The listing builds one solid part. Answer for the finished solid, in the listing's coordinates (mm). A direction names the side the tool comes from. Coordinates: 2 decimals unless noted, no trailing zeros. Loops run counter-clockwise (first coordinate to the right, second up) from the corner with the lowest first, then second, coordinate; pieces in that order, holes last. Notation, with made-up numbers: (79.5, 8) - (105.5, 8) arc R25 ccw to (105.5, 41) - close; hole circle Ø9 at (65.25, 12.5). An arc over 180 degrees is marked (long way). Return JSON: item names as keys, results as strings. Group by question number.
1. Each of these flat-tipped pins is pushed along its axis until it touches: P1, Ø3, axis at y = 1, z = 4, coming from the +X side; P2, Ø8, axis at x = 18.34, y = 0, coming from the +Z side; P3, Ø2, axis at x = 4.5, z = 5, coming from the +Y side; P4, Ø4, axis at x = 15.5, z = 4, coming from the -Y side. Where does it stop, or does it pass through?
2. Section B-B (z = 3) is taken. Write down the section's boundary in (x, y).
3. Section C-C (y = 0) is taken. Write down the section's boundary in (x, z).
4. The mould has two halves that part along X. Classify faces 3 (the face through (12.75, -7.76, 1.97)), 4 (the face through (-0.867, -3.905, 4.289)), 5 (the face through (-12.3, 4, 4)): pulls with the +X half, pulls with the -X half, needs draft (parallel to the pull), parting line crosses it, or undercut.
5. Section A-A (x = 0) is taken. Write down the section's boundary in (y, z).
6. Section D-D (y = 6.75) is taken. Write down the section's boundary in (x, z), and give its area (3 significant figures).
7. Find the intervals of material crossed by line 1 along Y through (x, z) = (0, 4.5); line 2 along Y through (x, z) = (0, 3); line 3 along X through (y, z) = (1.5, 3), in increasing order.
8. Which of the six approach directions +Z, -Z, +X, -X, +Y, -Y give full straight-line access (tool end or side, diameter ignored) to faces 1 (the face through (-2.75, -12.4, 6.32)), 2 (the face through (-16.03, -0.96, 1.97))?
```python
from build123d import *

# Parameters (mm, degrees)
SKETCH_R      = 4
SKETCH_R_2    = 2.5
PAD_DEPTH     = 4
SKETCH001_R   = 12.7
SKETCH001_R_2 = 4
PAD001_DEPTH  = 4.7


with BuildPart() as part:
    # Sketch → Pad (new body)
    with BuildSketch(Plane.XY):
        with BuildLine():
            Line((-20.376172, -4.856123), (-3.731608, -12.439939))
            ThreePointArc((-3.731608, -12.439939), (0.235589, -13.246916), (4.155117, -12.233421))
            Line((4.155117, -12.233421), (21.579522, -3.164572))
            ThreePointArc((21.579522, -3.164572), (23.5, 0), (21.579522, 3.164572))
            Line((21.579522, 3.164572), (4.155117, 12.233421))
            ThreePointArc((4.155117, 12.233421), (0.235589, 13.246916), (-3.731608, 12.439939))
            Line((-3.731608, 12.439939), (-20.376172, 4.856123))
            ThreePointArc((-20.376172, 4.856123), (-23.5, 0), (-20.376172, -4.856123))
        make_face()
        Circle(SKETCH_R, mode=Mode.SUBTRACT)
        with Locations((-18.336439, 0)):
            Circle(SKETCH_R_2, mode=Mode.SUBTRACT)
        with Locations((18.336439, 0)):
            Circle(SKETCH_R_2, mode=Mode.SUBTRACT)
    extrude(amount=PAD_DEPTH)

    # Sketch001 → Pad001 (new body)
    with BuildSketch(Plane.XY.offset(4)):
        Circle(SKETCH001_R)
        Circle(SKETCH001_R_2, mode=Mode.SUBTRACT)
    extrude(amount=PAD001_DEPTH)


solid = part.part
```
The answers:
{
 "1": {"P1": "stops at x = 23.5", "P2": "stops at z = 4", "P3": "stops at y = 12.21", "P4": "stops at y = -7.37"},
 "2": {"outline": "(-20.38, -4.86) - (-3.73, -12.44) arc R9 ccw to (4.16, -12.23) - (21.58, -3.16) arc R3.57 ccw to (21.58, 3.16) - (4.16, 12.23) arc R9 ccw to (-3.73, 12.44) - (-20.38, 4.86) arc R5.34 ccw to start; hole circle Ø5 at (-18.34, 0); hole circle Ø8 at (0, 0); hole circle Ø5 at (18.34, 0)"},
 "3": {"outline": "(-23.5, 0) - (-20.84, 0) - (-20.84, 4) - (-23.5, 4) - close; (-15.84, 0) - (-4, 0) - (-4, 8.7) - (-12.7, 8.7) - (-12.7, 4) - (-15.84, 4) - close; (4, 0) - (15.84, 0) - (15.84, 4) - (12.7, 4) - (12.7, 8.7) - (4, 8.7) - close; (20.84, 0) - (23.5, 0) - (23.5, 4) - (20.84, 4) - close"},
 "4": {"face 3": "pulls with the +X half", "face 4": "undercut", "face 5": "needs draft"},
 "5": {"outline": "(-13.25, 0) - (-4, 0) - (-4, 8.7) - (-12.7, 8.7) - (-12.7, 4) - (-13.25, 4) - close; (4, 0) - (13.25, 0) - (13.25, 4) - (12.7, 4) - (12.7, 8.7) - (4, 8.7) - close"},
 "6": {"outline": "(-16.22, 0) - (14.69, 0) - (14.69, 4) - (10.76, 4) - (10.76, 8.7) - (-10.76, 8.7) - (-10.76, 4) - (-16.22, 4) - close", "area": "225 mm2"},
 "7": {"line 1": "y = -12.7 to -4, 4 to 12.7", "line 2": "y = -13.25 to -4, 4 to 13.25", "line 3": "x = -23.28 to -20.34, -16.34 to -3.71, 3.71 to 16.34, 20.34 to 23.17"},
 "8": {"face 1": "+Z", "face 2": "+Z, -Z"}
}
